Verification items for the finished model (mm, model axes). Coordinates: 2 decimals unless noted, no trailing zeros. Order: outer loops, then holes, each group sorted by start corner. A loop starts at its lowest first (then second) coordinate and runs counter-clockwise, first axis right, second up. Notation, with made-up numbers: M 70,56 L 127,56 A27 ccw 127,91 Z; hole C 48.5,29 d1. An arc over 180 degrees is marked long. Return JSON: item names as keys, results as strings.
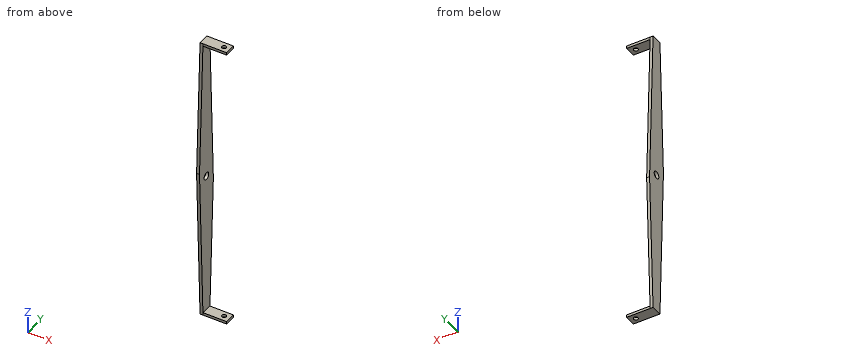
```python
from build123d import *

# Parameters (mm, degrees)
BOSS_EXTRUDE2_DEPTH = 2
SKETCH4_W           = 3.5
SKETCH4_H           = 15
BOSS_EXTRUDE3_DEPTH = 32
SKETCH5_R           = 3
CUT_EXTRUDE1_DEPTH  = 392
SKETCH7_R           = 5
CUT_EXTRUDE2_DEPTH  = 5


with BuildPart() as part:
    # Sketch2 → Boss-Extrude2 (new, symmetric)
    with BuildSketch(Plane(origin=(0, 0, 0), x_dir=(0, 0, -1), z_dir=(1, 0, 0))):
        Polygon((0, 0), (208, 7.5), (392, 0), (392, -15), (184, -22.5), (0, -15), align=None)
    extrude(amount=BOSS_EXTRUDE2_DEPTH, both=True)

    # Sketch4 → Boss-Extrude3 (add)
    with BuildSketch(Plane(origin=(2, 0, 0), x_dir=(0, 0, -1), z_dir=(1, 0, 0))):
        with Locations((1.75, -7.5)):
            Rectangle(SKETCH4_W, SKETCH4_H)
        with Locations((390.25, -7.5)):
            Rectangle(SKETCH4_W, SKETCH4_H)
    extrude(amount=BOSS_EXTRUDE3_DEPTH)

    # Sketch5 → Cut-Extrude1 (cut)
    with BuildSketch(Plane.XY):
        with Locations((26, -7.5)):
            Circle(SKETCH5_R)
    extrude(amount=-CUT_EXTRUDE1_DEPTH, mode=Mode.SUBTRACT)

    # Sketch7 → Cut-Extrude2 (cut)
    with BuildSketch(Plane.ZY.offset(2)):
        with Locations((-196, -7.5)):
            Circle(SKETCH7_R)
    extrude(amount=-CUT_EXTRUDE2_DEPTH, mode=Mode.SUBTRACT)


solid = part.part
```
Q1. Cross-section at A-A, the plane x = 10. Record the boundary of the cut face in (y, z).
Values:
{"outline": "M -15,-392 L 0,-392 L 0,-388.5 L -15,-388.5 Z; M -15,-3.5 L 0,-3.5 L 0,0 L -15,0 Z"}
Q2. Go/stop test with flat-tipped pins: pin 1 (1 mm diameter, centred on y = -11.5, z = -120, fed in from +X); pin 2 (5 mm diameter, centred on x = 25.5, y = -19, fed in from -Z); pin 3 (1 mm diameter, centred on x = 21.5, z = -2.5, fed in from -Y); pin 4 (3 mm diameter, centred on x = 11, z = -1, fed in from +Y). Record where each tip stops, or that it passes through.
Values:
{"pin 1": "x = 2", "pin 2": "through", "pin 3": "y = -15", "pin 4": "y = 0"}
Q3. Cross-section at C-C, the plane y = -19.25. Record the boundary of the cut face in (x, z), and give its area (3 significant figures).
Values:
{"outline": "M -2,-274.13 L 2,-274.13 L 2,-104.27 L -2,-104.27 Z", "area": "679 mm^2"}
Q4. Material ranges on line 1 along Z through (x, y) = (22.5, -8.5); line 2 along Y through (x, z) = (26, -1.2); line 3 along X through (y, z) = (-7, -38), recorded low to high.
Values:
{"line 1": "-392 to -388.5, -3.5 to 0", "line 2": "-15 to -10.5, -4.5 to 0", "line 3": "-2 to 2"}
Q5. Cross-section at D-D, the plane z = -237. Record the boundary of the cut face in (x, y), and give its area (3 significant figures).
Values:
{"outline": "M -2,-20.59 L 2,-20.59 L 2,6.32 L -2,6.32 Z", "area": "108 mm^2"}
Q6. Cross-section at B-B, the plane z = -196. Record the boundary of the cut face in (x, y).
Values:
{"outline": "M -2,-22.07 L 2,-22.07 L 2,-12.5 L -2,-12.5 Z; M -2,-2.5 L 2,-2.5 L 2,7.07 L -2,7.07 Z"}
